Geometry: final body of the model. Coordinates: model frame, mm. Face numbers are marked on the shaded views. A direction names the side the tool comes from. Round coordinates to 2 decimals unless told otherwise and drop trailing zeros. Write each loop counter-clockwise with the first axis right and the second up, starting at its lowest first coordinate (ties: lowest second). Pieces come first, ordered by that corner, then holes. Notation, with made-up numbers: (81, 38.25) -> (85, 38.25) arc R11 ccw to (85, 49.25) -> close; hole circle Ø10 at (68.5, 16.5). An arc over 180 degrees is marked (long way). Use one line per item in the form item = value. Start each with the question number.
1. Draft query along X for the marked faces 1, 2 and 3. Return one class per face: pulls with the +X half, pulls with the -X half, needs draft (parallel to the pull), parting line crosses it, or undercut.
2. Cut plane B-B, the plane y = 5.75. State how many separate pieces and enclosed holes the cut face has, plus the area to 3 significant figures.
3. Reachability of the marked faces 4 and 5 from +Z, -Z, +X, -X, +Y, -Y: full face, straight path, thin tool, end or side. Return the list, or none.
4. Line query: L1, parallel to X at y = 1.85, z = 0; L2, parallel to X at y = 2, z = -1; L3, parallel to Z at x = 0.75, y = 4.5. Output: solid intervals per line, ascending.
5. Pin query (flat end, axial travel): pin 1 Ø1.5 at (y, z) = (3.5, 2.5) entering from -X. Return the tip coordinate at first contact, or that it passes through.
6. Cut plane D-D, the plane x = -4. Return the cut outline in (y, z) (3 decimals).
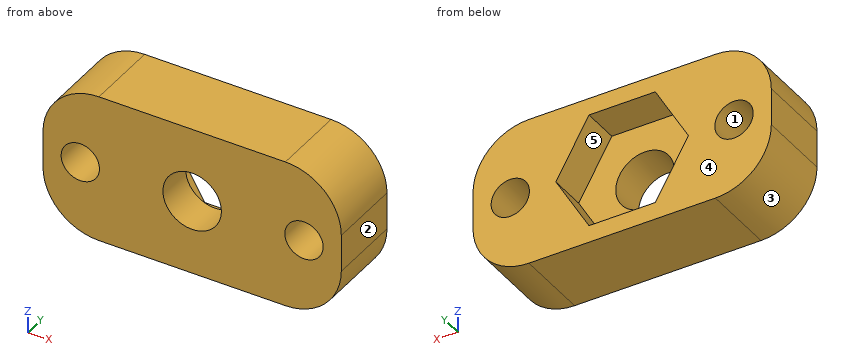
```python
from build123d import *

# Parameters (mm, degrees)
SKETCH1_W           = 25.4
SKETCH1_H           = 12.7
SKETCH1_R           = 1.63195
SKETCH1_R_2         = 2.4892
BOSS_EXTRUDE1_DEPTH = 3.175
SKETCH1_3_W         = 25.4
SKETCH1_3_H         = 12.7
SKETCH1_3_R         = 1.63195
BOSS_EXTRUDE2_DEPTH = 6.35
FILLET1_R           = 4.7625


with BuildPart() as part:
    # Sketch1 → Boss-Extrude1 (new body)
    # profile 1 of 2: a face of its own
    with BuildSketch(Plane(origin=(0, 0, 0), x_dir=(1, 0, 0), z_dir=(0, 1, 0))):
        Rectangle(SKETCH1_W, SKETCH1_H)
        with Locations(Location((9.525, 0, 0), (0, 0, 270))):
            Circle(SKETCH1_R, mode=Mode.SUBTRACT)
        with Locations(Location((-9.525, 0, 0), (0, 0, 270))):
            Circle(SKETCH1_R, mode=Mode.SUBTRACT)
        Polygon((2.822954141, -4.8895), (5.645908282, 0), (2.822954141, 4.8895), (-2.822954141, 4.8895), (-5.645908282, 0), (-2.822954141, -4.8895), align=None, mode=Mode.SUBTRACT)
    # profile 2 of 2: a face of its own
    with BuildSketch(Plane(origin=(0, 0, 0), x_dir=(1, 0, 0), z_dir=(0, 1, 0))):
        Polygon((-2.822954141, -4.8895), (2.822954141, -4.8895), (5.645908282, 0), (2.822954141, 4.8895), (-2.822954141, 4.8895), (-5.645908282, 0), align=None)
        with Locations(Location((0, 0, 0), (0, 0, 270))):
            Circle(SKETCH1_R_2, mode=Mode.SUBTRACT)
    extrude(amount=BOSS_EXTRUDE1_DEPTH)

    # Sketch1<3> → Boss-Extrude2 (add)
    with BuildSketch(Plane(origin=(0, 0, 0), x_dir=(1, 0, 0), z_dir=(0, 1, 0))):
        Rectangle(SKETCH1_3_W, SKETCH1_3_H)
        with Locations(Location((9.525, 0, 0), (0, 0, 270))):
            Circle(SKETCH1_3_R, mode=Mode.SUBTRACT)
        with Locations(Location((-9.525, 0, 0), (0, 0, 270))):
            Circle(SKETCH1_3_R, mode=Mode.SUBTRACT)
        Polygon((2.822954141, -4.8895), (5.645908282, 0), (2.822954141, 4.8895), (-2.822954141, 4.8895), (-5.645908282, 0), (-2.822954141, -4.8895), align=None, mode=Mode.SUBTRACT)
    extrude(amount=BOSS_EXTRUDE2_DEPTH)

    # Fillet1
    fillet1_edges = [part.edges().sort_by_distance(p)[0] for p in [
        (12.7, 3.175, 6.35),
        (-12.7, 3.175, 6.35),
        (-12.7, 3.175, -6.35),
        (12.7, 3.175, -6.35),
    ]]
    fillet(fillet1_edges, radius=FILLET1_R)


solid = part.part
```
Outcome:
q1.face_1 = undercut
q1.face_2 = pulls with the +X half
q1.face_3 = pulls with the -X half
q2.separate_pieces = 1
q2.enclosed_holes = 3
q2.area = 204 mm^2
q3.face_4 = +Z, -Z, +X, -X, +Y
q3.face_5 = +Y
q4.L1 = -12.7 to -11.16, -7.89 to -2.49, 2.49 to 7.89, 11.16 to 12.7
q4.L2 = -12.7 to -10.81, -8.24 to -2.28, 2.28 to 8.24, 10.81 to 12.7
q4.L3 = -6.35 to -4.89, 4.89 to 6.35
q5.pin_1 = -12.7
q6.outline = (0, -6.35) -> (6.35, -6.35) -> (6.35, -2.851) -> (3.175, -2.851) -> (3.175, 2.851) -> (6.35, 2.851) -> (6.35, 6.35) -> (0, 6.35) -> close
